from build123d import *

# Parameters (mm, degrees)
SKETCH_1_R      = 5.5
EXTRUDE_1_DEPTH = 3


with BuildPart() as part:
    # 草图1 → 凸台-拉伸1 (new body)
    with BuildSketch(Plane.XY):
        with BuildLine():
            Line((324.289682364, 18.881027034), (324.289682364, 433.044836172))
            Line((324.289682364, 433.044836172), (324.289682364, 445.746542094))
            Line((324.289682364, 445.746542094), (255.453360513, 485.489211044))
            ThreePointArc((255.453360513, 485.489211044), (240.427081072, 481.462931603), (244.453360513, 466.436652161))
            Line((244.453360513, 466.436652161), (296.41488474, 436.436652161))
            Line((296.41488474, 436.436652161), (296.41488474, 24.149465082))
            ThreePointArc((296.41488474, 24.149465082), (294.405265797, 16.649465082), (288.91488474, 11.159084025))
            Line((288.91488474, 11.159084025), (244.453360513, -14.510788956))
            ThreePointArc((244.453360513, -14.510788956), (240.427081072, -29.537068397), (255.453360513, -33.563347839))
            Line((255.453360513, -33.563347839), (316.789682364, 1.849194092))
            ThreePointArc((316.789682364, 1.849194092), (322.28006342, 7.339575149), (324.289682364, 14.839575149))
            Line((324.289682364, 14.839575149), (324.289682364, 18.881027034))
        make_face()
        with Locations((249.953360513, -24.037068397)):
            Circle(SKETCH_1_R, mode=Mode.SUBTRACT)
        with Locations((249.953360513, 475.962931603)):
            Circle(SKETCH_1_R, mode=Mode.SUBTRACT)
    extrude(amount=EXTRUDE_1_DEPTH)


solid = part.part
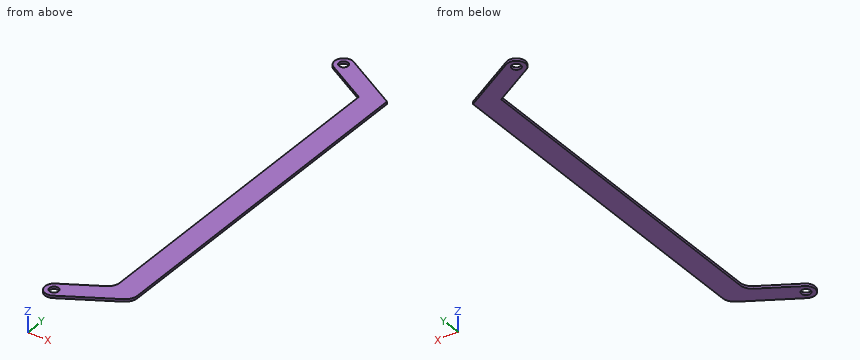
The listing builds one solid part. Answer for the finished solid, in the listing's coordinates (mm). Coordinates: 2 decimals unless noted, no trailing zeros. Order: outer loops, then holes, each group sorted by start corner. A loop starts at its lowest first (then second) coordinate and runs counter-clockwise, first axis right, second up.
Q1. A cutting plane is placed at C-C, the plane y = 73. Write down the section's boundary in (x, z).
Q2. A cutting plane is placed at A-A, the plane x = 280.5. Write down the section's boundary in (y, z).
Q3. A cutting plane is placed at B-B, the plane z = 0.9. Write down the section's boundary in (x, y), and give its area (3 significant figures).
Q4. A cutting plane is placed at D-D, the plane x = 307.5. Write down the section's boundary in (y, z).
Q5. Given P1, Ø17.5, axis at x = 249.95, y = -24.04, coming from the -Z side; P2, Ø1.5, axis at x = 293, z = 1.5, coming from the -Y side; P3, Ø1.5, axis at y = 361, z = 1.5, coming from the -X side; P4, Ø6.5, axis at x = 249.95, y = 475.96, coming from the +Z side, each flat-ended and moving along its own axis, determine where each tip first touches the part or whether it passes through.
Q6. Consider line 1 (Y direction, x = 251.5, z = 1.3); line 2 (Y direction, x = 246.5, z = 1.2); line 3 (X direction, y = 187.5, z = 2.8). Determine where each line is inside the solid, lowest interval first.
Answers follow:
1. outline: (296.41, 0) - (324.29, 0) - (324.29, 3) - (296.41, 3) - close
2. outline: (-19.1, 0) - (6.3, 0) - (6.3, 3) - (-19.1, 3) - close; (445.63, 0) - (471.03, 0) - (471.03, 3) - (445.63, 3) - close
3. outline: (244.45, -14.51) arc R11 ccw to (255.45, -33.56) - (316.79, 1.85) arc R15 ccw to (324.29, 14.84) - (324.29, 445.75) - (255.45, 485.49) arc R11 ccw to (244.45, 466.44) - (296.41, 436.44) - (296.41, 24.15) arc R15 cw to (288.91, 11.16) - close; hole circle Ø11 at (249.95, -24.04); hole circle Ø11 at (249.95, 475.96)
3. area: 15,300 mm2
4. outline: (-3.51, 0) - (455.44, 0) - (455.44, 3) - (-3.51, 3) - close
5. P1: stops at z = 0
5. P2: stops at y = -12.32
5. P3: stops at x = 296.41
5. P4: passes through
6. line 1: y = -34.93 to -29.32, -18.76 to -10.44, 462.37 to 470.68, 481.24 to 486.85
6. line 2: y = -34.48 to -28.32, -19.76 to -13.33, 465.26 to 471.68, 480.24 to 486.41
6. line 3: x = 296.41 to 324.29
